For this review, use the dimensioned drawing (mm, ordinates from the lowest corner) and the shaded views. A direction names the side the tool comes from. Coordinates: 2 decimals unless noted, no trailing zeros. Loops run counter-clockwise (first coordinate to the right, second up) from the corner with the lowest first, then second, coordinate; pieces in that order, holes last. Notation, with made-up numbers: M 59.5,79.25 L 107.5,79.25 A29 ccw 107.5,102.25 Z; hole C 21.25,-32.75 d10. An arc over 180 degrees is marked long. One line per item, written item: value.
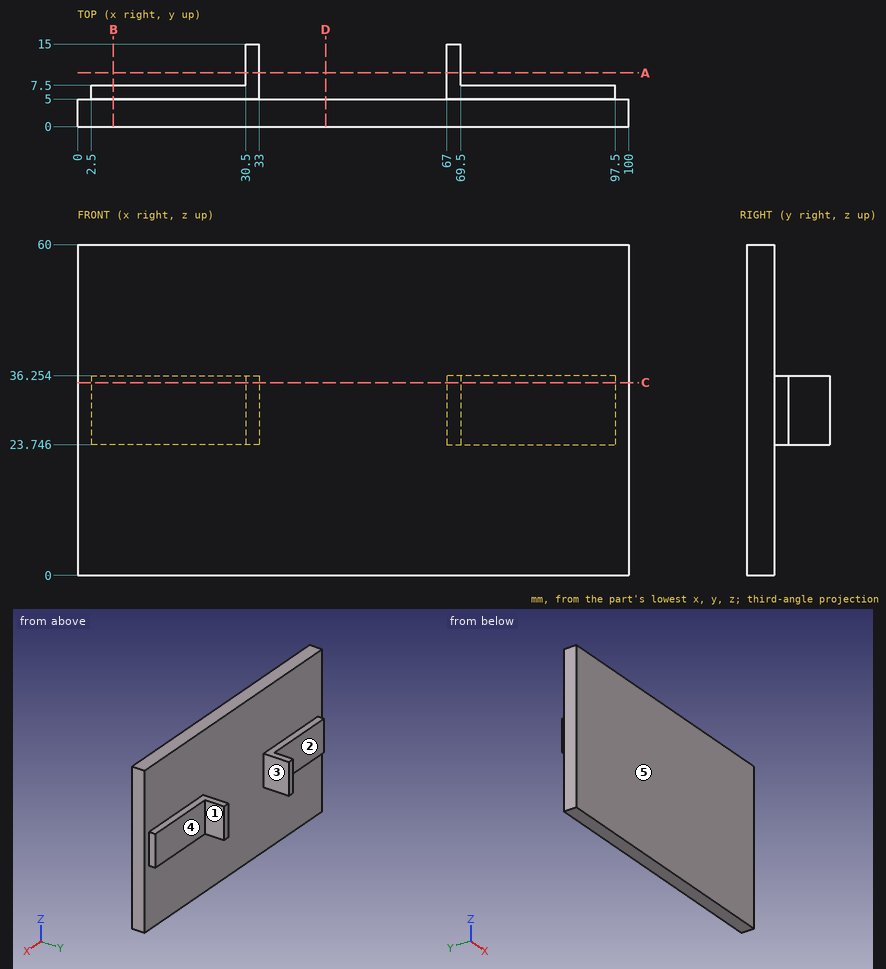
(1) Add section A-A on y = 9.75. State the section outline as (x, z) points, then the cut area to 3 significant figures.
Checks:
outline: M 30.5,23.75 L 33,23.75 L 33,36.25 L 30.5,36.25 Z; M 67,23.75 L 69.5,23.75 L 69.5,36.25 L 67,36.25 Z
area: 62.5 mm^2
(2) Add section B-B on x = 6.5. State the section outline as (y, z) points, then the cut area to 3 significant figures.
Checks:
outline: M 0,0 L 5,0 L 5,23.75 L 7.5,23.75 L 7.5,36.25 L 5,36.25 L 5,60 L 0,60 Z
area: 331 mm^2
(3) To check wall thickness, follow L1, parallel to X at y = 6.25, z = 24.5; L2, parallel to X at y = 9.75, z = 27.5; L3, parallel to Y at x = 32.5, z = 20. State the ranges of each line that lie inside material, in increasing order. Write a range as [from, to].
Checks:
L1: [2.5, 33], [67, 97.5]
L2: [30.5, 33], [67, 69.5]
L3: [0, 5]
(4) Insertion check: pin 1 Ø4 at (x, z) = (78, 27.5) entering from +Y; pin 2 Ø10 at (x, z) = (79, 52) entering from +Y; pin 3 Ø5 at (x, y) = (18, 8.5) entering from -Z; pin 4 Ø5 at (x, y) = (81, 12) entering from +Z. Each pin has a flat end and moves straight along its axis. Give the tip position at first contact, or say it passes through.
Checks:
pin 1: y = 7.5
pin 2: y = 5
pin 3: z = 23.75
pin 4: through
(5) Add section C-C on z = 35. State the section outline as (x, y) points.
Checks:
outline: M 0,0 L 100,0 L 100,5 L 97.5,5 L 97.5,7.5 L 69.5,7.5 L 69.5,15 L 67,15 L 67,5 L 33,5 L 33,15 L 30.5,15 L 30.5,7.5 L 2.5,7.5 L 2.5,5 L 0,5 Z
(6) Tool access review of the marked faces 4 and 5: name each direction out of +Z, -Z, +X, -X, +Y, -Y from which nothing blocks a thin tool from reaching the whole face with its end or side.
Checks:
face 4: +Z, -Z, +X, +Y
face 5: +Z, -Z, +X, -X, -Y
(7) Draft analysis for pull direction X (two halves, no side actions). For the marked faces 1, 2 and 3, state which applies: pulls with the +X half, pulls with the -X half, needs draft (parallel to the pull), parting line crosses it, or undercut.
Checks:
face 1: pulls with the +X half
face 2: needs draft
face 3: undercut
(8) Add section D-D on x = 45. State the section outline as (y, z) points.
Checks:
outline: M 0,0 L 5,0 L 5,60 L 0,60 Z
